The listing builds one solid part. Answer for the finished solid, in the listing's coordinates (mm). A direction names the side the tool comes from. Round coordinates to 2 decimals unless told otherwise and drop trailing zeros. Write each loop counter-clockwise with the first axis right and the second up, starting at its lowest first coordinate (ties: lowest second). Pieces come first, ordered by that corner, then holes.
Item 1: A tool of negligible diameter and unlimited length cuts with its end or side. For faces 1 (the face through (14, -90, 11)), 2 (the face through (27.4, -68.568, 12.7)), 3 (the face through (11.447, -79.132, 16.987)), 4 (the face through (26.23, -64.17, 24.63)), 5 (the face through (22, -99.768, 3)), from which of +Z, -Z, +X, -X, +Y, -Y can it reach the whole face along a straight path? Write none if from no direction.
Item 2: For a pull along X with two mould halves and no side action, classify faces 6 (the face through (14, -79.703, 18)), 7 (the face through (28.92, -81.79, 2.46)), 8 (the face through (15.846, -80.5, 10.8)) as +X half, -X half, draft (parallel to the pull), parting line (faces both ways), or undercut.
Item 3: Find section C-C on x = 33. Give the vertices of the cut face in (y, z).
Item 4: Find the intervals of material crossed by probe 1 along X at (y, z) = (-66.1, 15.2); probe 2 along Z at (x, y) = (21.25, -96.5); probe 3 along Y at (x, z) = (31.25, 7), in increasing order.
Item 5: Find section D-D on z = 8. Give the vertices of the cut face in (x, y).
Item 6: Find section B-B on y = -73. Give the vertices of the cut face in (x, z).
Item 7: Each of these flat-tipped pins is pushed along its axis until it touches: pin 1 (0.9 mm diameter, centred on x = 15, y = -92, fed in from +Z); pin 2 (10 mm diameter, centred on y = -80.5, z = 10.5, fed in from +X); pin 3 (12 mm diameter, centred on x = 33, y = -90.5, fed in from +Z). Where does it stop, or does it pass through?
Item 8: Find section A-A on z = 15.2. Give the vertices of the cut face in (x, y).
```python
from build123d import *

# Parameters (mm, degrees)
ESQUISSE1_W        = 23.4
ESQUISSE1_H        = 31.2
ESQUISSE1_R        = 2.5
BOSS_EXTRU_1_DEPTH = 5
ESQUISSE3_W        = 23.4
ESQUISSE3_H        = 25.2
ESQUISSE3_R        = 2.5
BOSS_EXTRU_3_DEPTH = 5
BOSS_EXTRU_2_DEPTH = 5
CONG_1_R           = 2


with BuildPart() as part:
    # Esquisse1 → Boss.-Extru.1 (new body)
    with BuildSketch(Plane.XY):
        with Locations((27.545883061, -84.168430722)):
            Rectangle(ESQUISSE1_W, ESQUISSE1_H)
        with Locations((29.245883061, -84.268430722)):
            Circle(ESQUISSE1_R, mode=Mode.SUBTRACT)
    extrude(amount=BOSS_EXTRU_1_DEPTH)

    # Esquisse3 → Boss.-Extru.3 (add)
    with BuildSketch(Plane(origin=(0, -68.568430722, 0), x_dir=(1, 0, 0), z_dir=(0, 1, 0))):
        with Locations((27.545883061, -12.6)):
            Rectangle(ESQUISSE3_W, ESQUISSE3_H)
        with Locations(Location((26.045883061, -15.2, 0), (0, 0, 270))):
            Circle(ESQUISSE3_R, mode=Mode.SUBTRACT)
    extrude(amount=BOSS_EXTRU_3_DEPTH)

    # Esquisse2 → Boss.-Extru.2 (add)
    with BuildSketch(Plane(origin=(15.845883061, 0, 12.450490199), x_dir=(0, 0, -1), z_dir=(1, 0, 0))):
        Polygon((12.450490199, -99.768430722), (12.450490199, -63.568430722), (-12.749509801, -63.568430722), (-12.749509801, -79.702669736), (1.450490199, -79.702669736), (1.450490199, -99.768430722), align=None)
    extrude(amount=-BOSS_EXTRU_2_DEPTH)

    # Congé1
    cong_1_edges = [part.edges().sort_by_distance(p)[0] for p in [
        (25.045883061, -63.568430722, 25.2),
        (39.245883061, -63.568430722, 12.6),
        (25.045883061, -63.568430722, 0),
        (10.845883061, -89.735550229, 11),
        (10.845883061, -79.702669736, 18.1),
        (10.845883061, -71.635550229, 25.2),
        (10.845883061, -63.568430722, 12.6),
        (10.845883061, -81.668430722, 0),
        (39.245883061, -81.668430722, 0),
    ]]
    fillet(cong_1_edges, radius=CONG_1_R)


solid = part.part
```
Check values:
1. face 1: +Z, +X, -X, -Y
1. face 2: +Z, +X, -Y
1. face 3: +Z, -X, -Y
1. face 4: +Z, +X, -X, +Y
1. face 5: +Z, -Z, +X, -X, -Y
2. face 6: draft
2. face 7: undercut
2. face 8: +X half
3. outline: (-99.77, 0) - (-65.57, 0) arc R2 ccw to (-63.57, 2) - (-63.57, 23.2) arc R2 ccw to (-65.57, 25.2) - (-68.57, 25.2) - (-68.57, 5) - (-99.77, 5) - close
4. probe 1: x = 10.85 to 23.55, 28.55 to 39.25
4. probe 2: z = 0 to 5
4. probe 3: y = -68.57 to -63.57
5. outline: (10.85, -99.77) - (15.85, -99.77) - (15.85, -68.57) - (39.25, -68.57) - (39.25, -65.57) arc R2 ccw to (37.25, -63.57) - (12.85, -63.57) arc R2 ccw to (10.85, -65.57) - close
6. outline: (10.85, 2) arc R2 ccw to (12.85, 0) - (37.25, 0) arc R2 ccw to (39.25, 2) - (39.25, 5) - (15.85, 5) - (15.85, 25.2) - (12.85, 25.2) arc R2 ccw to (10.85, 23.2) - close
7. pin 1: stops at z = 11
7. pin 2: stops at x = 15.85
7. pin 3: stops at z = 5
8. outline: (10.85, -77.7) arc R2 ccw to (12.85, -79.7) - (15.85, -79.7) - (15.85, -68.57) - (23.55, -68.57) - (23.55, -63.57) - (12.85, -63.57) arc R2 ccw to (10.85, -65.57) - close; (28.55, -68.57) - (39.25, -68.57) - (39.25, -65.57) arc R2 ccw to (37.25, -63.57) - (28.55, -63.57) - close
